Drawing for the job (mm, zero at the part's lowest x, y, z). A direction names the side the tool comes from. Coordinates: 2 decimals unless noted, no trailing zeros. Order: outer loops, then holes, each group sorted by start corner. A loop starts at its lowest first (then second) coordinate and runs counter-clockwise, first axis right, second up.
1) Cut at A-A (z = 26.5). List the corners of the cut face in (x, y).
2) Wall check: L1, parallel to Y at x = 134.5, z = 6; L2, parallel to X at y = 5, z = 10. Give the ranges that are in metal, low to high.
3) Pin check, flat tips, straight feed: pin 1 Ø10 at (x, y) = (85, 26) entering from -Z; pin 2 Ø4 at (y, z) = (10, 58.5) entering from +X; pin 3 Ø3 at (x, z) = (22, 41.5) entering from -Y; pin 4 Ø6 at (x, y) = (124.5, 33.5) entering from -Z. Stop position of each tip, or through.
4) Cut at B-B (x = 76.5). List the corners of the cut face in (y, z).
5) Cut at C-C (y = 14). List the corners of the cut face in (x, z), and give its area (3 significant figures).
6) Tool access for the marked faces 1 and 2: list every direction of +Z, -Z, +X, -X, +Y, -Y with a clear straight run to the whole face (end or side of a thin tool).
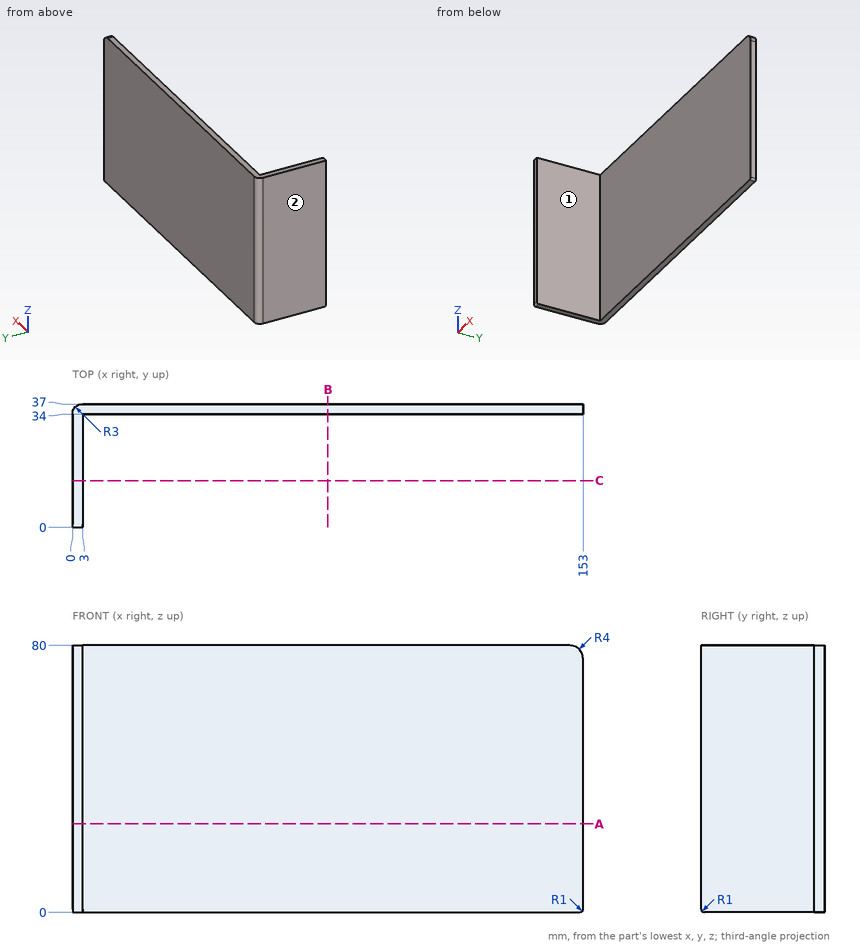
Geometry check:
1. outline: (0, 0) - (3, 0) - (3, 34) - (153, 34) - (153, 37) - (3, 37) arc R3 ccw to (0, 34) - close
2. L1: y = 34 to 37
2. L2: x = 0 to 3
3. pin 1: passes through
3. pin 2: stops at x = 3
3. pin 3: stops at y = 34
3. pin 4: stops at z = 0
4. outline: (34, 0) - (37, 0) - (37, 80) - (34, 80) - close
5. outline: (0, 0) - (3, 0) - (3, 80) - (0, 80) - close
5. area: 240 mm2
6. face 1: +Z, -Z, +X, -Y
6. face 2: +Z, -Z, -X, +Y, -Y
